Build history of the part. All positions in model axes, mm. Face numbers are marked on the shaded views. A direction names the side the tool comes from. Round coordinates to 2 decimals unless told otherwise and drop trailing zeros. Write each loop counter-clockwise with the first axis right and the second up, starting at its lowest first coordinate (ties: lowest second). Pieces come first, ordered by that corner, then holes.
1) Saw through at A-A (x = 7). Write the cut outline in (y, z), plus the area to 3 significant figures.
2) Flat gauge pins, fed straight in: pin 1 (1 mm diameter, centred on x = 38, y = -12.5, fed in from +Z); pin 2 (8 mm diameter, centred on x = 18.5, z = -44, fed in from +Y); pin 3 (4 mm diameter, centred on x = 16, z = -23, fed in from -Y); pin 4 (5 mm diameter, centred on x = 7.5, y = -8, fed in from -Z). Where does each tip first touch, or does it go through?
3) Saw through at C-C (z = -13). Write the cut outline in (x, y), plus the area to 3 significant figures.
4) Pull direction Z, two halves, no side cores. Call the marked faces 4, 5 and 6: +Z half, -Z half, draft (parallel to the pull), parting line (faces both ways), or undercut.
5) Wall check: probe 1 along X at (y, z) = (11, -25); probe 2 along X at (y, z) = (-7, -3); probe 3 along Y at (x, z) = (31.55, -6). Give the ranges that are in metal, low to high.
6) Saw through at B-B (y = -6.5). Write the cut outline in (x, z), plus the area to 3 significant figures.
7) Which spindle directions (+Z, -Z, +X, -X, +Y, -Y) get a long thin tool onto all of the face, cutting with end or side? Do the marked faces 1, 2 and 3. Say none if no direction does.
8) Saw through at D-D (y = 3). Write the cut outline in (x, z), plus the area to 3 significant figures.
from build123d import *

# Parameters (mm, degrees)
BOSS_EXTRUDE1_DEPTH   = 6
SKETCH16_R            = 4.5
BOSS_EXTRUDE3_DEPTH   = 12
SKETCH16_3_R          = 4.5
BOSS_EXTRUDE4_DEPTH   = 2
CUT_EXTRUDE1_DEPTH    = 4.5
F_5_4MM_DOWEL_HOLE1_D = 5.4
F_7_4MM_DOWEL_HOLE2_D = 7.4
SKETCH2_W             = 6
SKETCH2_H             = 12
BOSS_EXTRUDE2_DEPTH   = 20
F_5_4MM_DOWEL_HOLE3_D = 5.4
FILLET1_R             = 6


with BuildPart() as part:
    # Sketch1 → Boss-Extrude1 (new body)
    with BuildSketch(Plane(origin=(0, 0, 0), x_dir=(1, 0, 0), z_dir=(0, 1, 0))):
        Polygon((40, 5.65), (40, 0), (0, 0), (0, 53), (40, 53), (40, 13.65), (44, 13.65), (44, 5.65), align=None)
    extrude(amount=BOSS_EXTRUDE1_DEPTH)

    # Sketch16 → Boss-Extrude3 (add)
    with BuildSketch(Plane(origin=(0, 6, 0), x_dir=(1, 0, 0), z_dir=(0, 1, 0))):
        with Locations((16, 25)):
            Circle(SKETCH16_R)
    extrude(amount=BOSS_EXTRUDE3_DEPTH)

    # Sketch16<3> → Boss-Extrude4 (add)
    with BuildSketch(Plane(origin=(0, 6, 0), x_dir=(1, 0, 0), z_dir=(0, 1, 0))):
        with Locations((24, 13)):
            Circle(SKETCH16_3_R)
    extrude(amount=BOSS_EXTRUDE4_DEPTH)

    # Sketch12 → Cut-Extrude1 (cut)
    with BuildSketch(Plane.XZ):
        Polygon((28.2, -10.575128869), (24, -8.150257739), (19.8, -10.575128869), (19.8, -15.424871131), (24, -17.849742261), (28.2, -15.424871131), align=None)
        Polygon((16, -20.150257739), (11.8, -22.575128869), (11.8, -27.424871131), (16, -29.849742261), (20.2, -27.424871131), (20.2, -22.575128869), align=None)
    extrude(amount=-CUT_EXTRUDE1_DEPTH, mode=Mode.SUBTRACT)

    # Ø5.4mm Dowel Hole1 (through all)
    with Locations(Plane(origin=(0, 0, 0), x_dir=(-1, 0, 0), z_dir=(0, -1, 0))):
        with Locations((-16, 25), (-24, 13)):
            Hole(F_5_4MM_DOWEL_HOLE1_D / 2)

    # Ø7.4mm Dowel Hole2 (through all)
    with Locations(Plane(origin=(0, 6, 0), x_dir=(1, 0, 0), z_dir=(0, 1, 0))):
        with Locations((7, 46)):
            f_7_4mm_dowel_hole2 = Hole(F_7_4MM_DOWEL_HOLE2_D / 2)

    # Sketch2 → Boss-Extrude2 (add)
    with BuildSketch(Plane.XZ):
        with Locations((6.8, -6)):
            Rectangle(SKETCH2_W, SKETCH2_H)
    boss_extrude2 = extrude(amount=BOSS_EXTRUDE2_DEPTH)

    # Ø5.4mm Dowel Hole3 (through all)
    with Locations(Plane(origin=(9.8, 0, 0), x_dir=(0, 0, -1), z_dir=(1, 0, 0))):
        with Locations((6, -10)):
            f_5_4mm_dowel_hole3 = Hole(F_5_4MM_DOWEL_HOLE3_D / 2)

    # Mirror1: Ø7.4mm Dowel Hole2, Boss-Extrude2, Ø5.4mm Dowel Hole3 across plane
    add(f_7_4mm_dowel_hole2.mirror(Plane(origin=(20, 0, 0), x_dir=(0, 0, 1), z_dir=(1, 0, 0))), mode=Mode.SUBTRACT)
    add(boss_extrude2.mirror(Plane(origin=(20, 0, 0), x_dir=(0, 0, 1), z_dir=(1, 0, 0))))
    add(f_5_4mm_dowel_hole3.mirror(Plane(origin=(20, 0, 0), x_dir=(0, 0, 1), z_dir=(1, 0, 0))), mode=Mode.SUBTRACT)

    # Fillet1
    fillet1_edges = [part.edges().sort_by_distance(p)[0] for p in [
        (0, 3, -53),
        (40, 3, -53),
    ]]
    fillet(fillet1_edges, radius=FILLET1_R)


solid = part.part
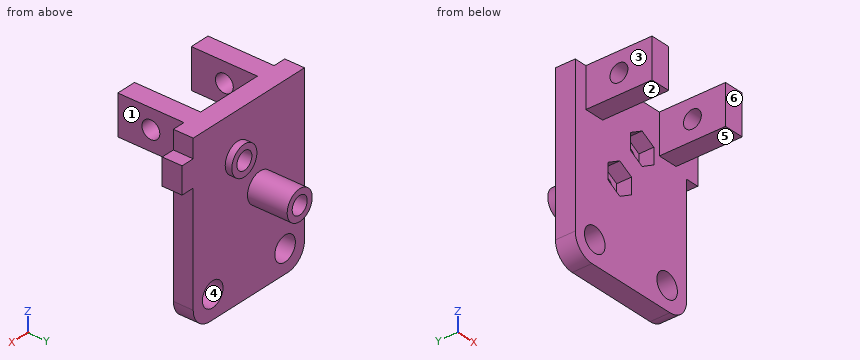
Evaluation:
1. outline: (-20, -12) - (0, -12) - (0, -42.3) - (6, -42.3) - (6, 0) - (-20, 0) - close; (0, -53) - (6, -53) - (6, -49.7) - (0, -49.7) - close; hole circle Ø5.4 at (-10, -6)
1. area: 491 mm2
2. pin 1: passes through
2. pin 2: stops at y = 6
2. pin 3: stops at y = 4.5
2. pin 4: stops at z = -12
3. outline: (0, 0) - (19.8, 0) - (19.8, 4.5) - (21.3, 4.5) - (21.3, 8) - (19.5, 8) - (19.5, 6) - (0, 6) - close; (26.7, 4.5) - (28.2, 4.5) - (28.2, 0) - (44, 0) - (44, 6) - (28.5, 6) - (28.5, 8) - (26.7, 8) - close
3. area: 225 mm2
4. face 4: undercut
4. face 5: -Z half
4. face 6: draft
5. probe 1: x = 11.5 to 13.3, 18.7 to 20.5
5. probe 2: x = 3.8 to 9.8, 30.2 to 36.2
5. probe 3: y = -20 to -12.7, -7.3 to 6
6. outline: (3.8, -12) - (9.8, -12) - (9.8, 0) - (3.8, 0) - close; (30.2, -12) - (36.2, -12) - (36.2, 0) - (30.2, 0) - close
6. area: 144 mm2
7. face 1: +Z, -Z, +X, -Y
7. face 2: -Z, +X, -X, -Y
7. face 3: +Z, -Z, -X, -Y
8. outline: (0, -47) arc R6 ccw to (6, -53) - (34, -53) arc R6 ccw to (40, -47) - (40, -13.65) - (44, -13.65) - (44, -5.65) - (40, -5.65) - (40, 0) - (0, 0) - close; hole circle Ø7.4 at (7, -46); hole (11.8, -27.42) - (16, -29.85) - (20.2, -27.42) - (20.2, -22.58) - (16, -20.15) - (11.8, -22.58) - close; hole (19.8, -15.42) - (24, -17.85) - (28.2, -15.42) - (28.2, -10.58) - (24, -8.15) - (19.8, -10.58) - close; hole circle Ø7.4 at (33, -46)
8. area: 1,930 mm2
